from build123d import *

# Parameters (mm, degrees)
PRISM_DEPTH       = 31
CYLINDER030_R     = 2.75
CYLINDER030_DEPTH = 6
CYLINDER029_R     = 5.2188
CYLINDER029_DEPTH = 31
CYLINDER007_R     = 8
CYLINDER007_DEPTH = 1.5
CYLINDER005_R     = 7.5
CYLINDER005_DEPTH = 2
CYLINDER011_R     = 8
CYLINDER011_DEPTH = 1.5
CYLINDER009_R     = 7.5
CYLINDER009_DEPTH = 2
CYLINDER015_R     = 8
CYLINDER015_DEPTH = 1.5
CYLINDER013_R     = 7.5
CYLINDER013_DEPTH = 2
CYLINDER019_R     = 8
CYLINDER019_DEPTH = 1.5
CYLINDER017_R     = 7.5
CYLINDER017_DEPTH = 2
CYLINDER023_R     = 8
CYLINDER023_DEPTH = 1.5
CYLINDER021_R     = 7.5
CYLINDER021_DEPTH = 2
CYLINDER027_R     = 8
CYLINDER027_DEPTH = 1.5
CYLINDER025_R     = 7.5
CYLINDER025_DEPTH = 2
CYLINDER003_R     = 8
CYLINDER003_DEPTH = 1.5
CYLINDER001_R     = 7.5
CYLINDER001_DEPTH = 2
CYLINDER_R        = 9
CYLINDER_DEPTH    = 4


with BuildPart() as prism:
    # prism → prism (new body)
    with BuildSketch(Plane.XY.offset(4)):
        Polygon((5.08068, 0), (2.54034, 4.399998), (-2.54034, 4.399998), (-5.08068, 0), (-2.54034, -4.399998), (2.54034, -4.399998), align=None)
    extrude(amount=PRISM_DEPTH)


with BuildPart() as cylinder030:
    # cylinder030 → cylinder030 (new body)
    with BuildSketch(Plane.XY.offset(-1)):
        Circle(CYLINDER030_R)
    extrude(amount=CYLINDER030_DEPTH)


with BuildPart() as union001:
    # cylinder029 → cylinder029 (new body)
    with BuildSketch(Plane.XY.offset(8)):
        Circle(CYLINDER029_R)
    extrude(amount=CYLINDER029_DEPTH)

    # union001: union prism, cylinder030
    add(prism.part)
    add(cylinder030.part)


with BuildPart() as cylinder006:
    # cylinder006 → cylinder006 (revolve)
    with BuildSketch(Plane(origin=(0, 0, 1.5), x_dir=(1, 0, 0), z_dir=(0, -1, 0))):
        Polygon((0, 0), (7.5, 0), (8, 0.5), (0, 0.5), align=None)
    revolve(axis=Axis((0, 0, 1.5), (0, 0, 1)))


with BuildPart() as cylinder007:
    # cylinder007 → cylinder007 (new body)
    with BuildSketch(Plane.XY.offset(2)):
        Circle(CYLINDER007_R)
    extrude(amount=CYLINDER007_DEPTH)


with BuildPart() as cylinder008:
    # cylinder008 → cylinder008 (revolve)
    with BuildSketch(Plane(origin=(0, 0, 3.5), x_dir=(1, 0, 0), z_dir=(0, -1, 0))):
        Polygon((0, 0), (8, 0), (7.5, 0.5), (0, 0.5), align=None)
    revolve(axis=Axis((0, 0, 3.5), (0, 0, 1)))


with BuildPart() as matrix_union001:
    # cylinder005 → cylinder005 (new body)
    with BuildSketch(Plane.XY):
        Circle(CYLINDER005_R)
    extrude(amount=CYLINDER005_DEPTH)

    # Matrix_Union001: union cylinder006, cylinder007, cylinder008
    add(cylinder006.part)
    add(cylinder007.part)
    add(cylinder008.part)


with BuildPart() as matrix_union001_1:
    # Matrix_Union001 placement: moved
    add(matrix_union001.part.moved(Location((0, 0, 4))))


with BuildPart() as cylinder010:
    # cylinder010 → cylinder010 (revolve)
    with BuildSketch(Plane(origin=(0, 0, 1.5), x_dir=(1, 0, 0), z_dir=(0, -1, 0))):
        Polygon((0, 0), (7.5, 0), (8, 0.5), (0, 0.5), align=None)
    revolve(axis=Axis((0, 0, 1.5), (0, 0, 1)))


with BuildPart() as cylinder011:
    # cylinder011 → cylinder011 (new body)
    with BuildSketch(Plane.XY.offset(2)):
        Circle(CYLINDER011_R)
    extrude(amount=CYLINDER011_DEPTH)


with BuildPart() as cylinder012:
    # cylinder012 → cylinder012 (revolve)
    with BuildSketch(Plane(origin=(0, 0, 3.5), x_dir=(1, 0, 0), z_dir=(0, -1, 0))):
        Polygon((0, 0), (8, 0), (7.5, 0.5), (0, 0.5), align=None)
    revolve(axis=Axis((0, 0, 3.5), (0, 0, 1)))


with BuildPart() as matrix_union002:
    # cylinder009 → cylinder009 (new body)
    with BuildSketch(Plane.XY):
        Circle(CYLINDER009_R)
    extrude(amount=CYLINDER009_DEPTH)

    # Matrix_Union002: union cylinder010, cylinder011, cylinder012
    add(cylinder010.part)
    add(cylinder011.part)
    add(cylinder012.part)


with BuildPart() as matrix_union002_1:
    # Matrix_Union002 placement: moved
    add(matrix_union002.part.moved(Location((0, 0, 8))))


with BuildPart() as cylinder014:
    # cylinder014 → cylinder014 (revolve)
    with BuildSketch(Plane(origin=(0, 0, 1.5), x_dir=(1, 0, 0), z_dir=(0, -1, 0))):
        Polygon((0, 0), (7.5, 0), (8, 0.5), (0, 0.5), align=None)
    revolve(axis=Axis((0, 0, 1.5), (0, 0, 1)))


with BuildPart() as cylinder015:
    # cylinder015 → cylinder015 (new body)
    with BuildSketch(Plane.XY.offset(2)):
        Circle(CYLINDER015_R)
    extrude(amount=CYLINDER015_DEPTH)


with BuildPart() as cylinder016:
    # cylinder016 → cylinder016 (revolve)
    with BuildSketch(Plane(origin=(0, 0, 3.5), x_dir=(1, 0, 0), z_dir=(0, -1, 0))):
        Polygon((0, 0), (8, 0), (7.5, 0.5), (0, 0.5), align=None)
    revolve(axis=Axis((0, 0, 3.5), (0, 0, 1)))


with BuildPart() as matrix_union003:
    # cylinder013 → cylinder013 (new body)
    with BuildSketch(Plane.XY):
        Circle(CYLINDER013_R)
    extrude(amount=CYLINDER013_DEPTH)

    # Matrix_Union003: union cylinder014, cylinder015, cylinder016
    add(cylinder014.part)
    add(cylinder015.part)
    add(cylinder016.part)


with BuildPart() as matrix_union003_1:
    # Matrix_Union003 placement: moved
    add(matrix_union003.part.moved(Location((0, 0, 12))))


with BuildPart() as cylinder018:
    # cylinder018 → cylinder018 (revolve)
    with BuildSketch(Plane(origin=(0, 0, 1.5), x_dir=(1, 0, 0), z_dir=(0, -1, 0))):
        Polygon((0, 0), (7.5, 0), (8, 0.5), (0, 0.5), align=None)
    revolve(axis=Axis((0, 0, 1.5), (0, 0, 1)))


with BuildPart() as cylinder019:
    # cylinder019 → cylinder019 (new body)
    with BuildSketch(Plane.XY.offset(2)):
        Circle(CYLINDER019_R)
    extrude(amount=CYLINDER019_DEPTH)


with BuildPart() as cylinder020:
    # cylinder020 → cylinder020 (revolve)
    with BuildSketch(Plane(origin=(0, 0, 3.5), x_dir=(1, 0, 0), z_dir=(0, -1, 0))):
        Polygon((0, 0), (8, 0), (7.5, 0.5), (0, 0.5), align=None)
    revolve(axis=Axis((0, 0, 3.5), (0, 0, 1)))


with BuildPart() as matrix_union004:
    # cylinder017 → cylinder017 (new body)
    with BuildSketch(Plane.XY):
        Circle(CYLINDER017_R)
    extrude(amount=CYLINDER017_DEPTH)

    # Matrix_Union004: union cylinder018, cylinder019, cylinder020
    add(cylinder018.part)
    add(cylinder019.part)
    add(cylinder020.part)


with BuildPart() as matrix_union004_1:
    # Matrix_Union004 placement: moved
    add(matrix_union004.part.moved(Location((0, 0, 16))))


with BuildPart() as cylinder022:
    # cylinder022 → cylinder022 (revolve)
    with BuildSketch(Plane(origin=(0, 0, 1.5), x_dir=(1, 0, 0), z_dir=(0, -1, 0))):
        Polygon((0, 0), (7.5, 0), (8, 0.5), (0, 0.5), align=None)
    revolve(axis=Axis((0, 0, 1.5), (0, 0, 1)))


with BuildPart() as cylinder023:
    # cylinder023 → cylinder023 (new body)
    with BuildSketch(Plane.XY.offset(2)):
        Circle(CYLINDER023_R)
    extrude(amount=CYLINDER023_DEPTH)


with BuildPart() as cylinder024:
    # cylinder024 → cylinder024 (revolve)
    with BuildSketch(Plane(origin=(0, 0, 3.5), x_dir=(1, 0, 0), z_dir=(0, -1, 0))):
        Polygon((0, 0), (8, 0), (7.5, 0.5), (0, 0.5), align=None)
    revolve(axis=Axis((0, 0, 3.5), (0, 0, 1)))


with BuildPart() as matrix_union005:
    # cylinder021 → cylinder021 (new body)
    with BuildSketch(Plane.XY):
        Circle(CYLINDER021_R)
    extrude(amount=CYLINDER021_DEPTH)

    # Matrix_Union005: union cylinder022, cylinder023, cylinder024
    add(cylinder022.part)
    add(cylinder023.part)
    add(cylinder024.part)


with BuildPart() as matrix_union005_1:
    # Matrix_Union005 placement: moved
    add(matrix_union005.part.moved(Location((0, 0, 20))))


with BuildPart() as cylinder026:
    # cylinder026 → cylinder026 (revolve)
    with BuildSketch(Plane(origin=(0, 0, 1.5), x_dir=(1, 0, 0), z_dir=(0, -1, 0))):
        Polygon((0, 0), (7.5, 0), (8, 0.5), (0, 0.5), align=None)
    revolve(axis=Axis((0, 0, 1.5), (0, 0, 1)))


with BuildPart() as cylinder027:
    # cylinder027 → cylinder027 (new body)
    with BuildSketch(Plane.XY.offset(2)):
        Circle(CYLINDER027_R)
    extrude(amount=CYLINDER027_DEPTH)


with BuildPart() as cylinder028:
    # cylinder028 → cylinder028 (revolve)
    with BuildSketch(Plane(origin=(0, 0, 3.5), x_dir=(1, 0, 0), z_dir=(0, -1, 0))):
        Polygon((0, 0), (8, 0), (7.5, 0.5), (0, 0.5), align=None)
    revolve(axis=Axis((0, 0, 3.5), (0, 0, 1)))


with BuildPart() as matrix_union006:
    # cylinder025 → cylinder025 (new body)
    with BuildSketch(Plane.XY):
        Circle(CYLINDER025_R)
    extrude(amount=CYLINDER025_DEPTH)

    # Matrix_Union006: union cylinder026, cylinder027, cylinder028
    add(cylinder026.part)
    add(cylinder027.part)
    add(cylinder028.part)


with BuildPart() as matrix_union006_1:
    # Matrix_Union006 placement: moved
    add(matrix_union006.part.moved(Location((0, 0, 24))))


with BuildPart() as cylinder002:
    # cylinder002 → cylinder002 (revolve)
    with BuildSketch(Plane(origin=(0, 0, 1.5), x_dir=(1, 0, 0), z_dir=(0, -1, 0))):
        Polygon((0, 0), (7.5, 0), (8, 0.5), (0, 0.5), align=None)
    revolve(axis=Axis((0, 0, 1.5), (0, 0, 1)))


with BuildPart() as cylinder003:
    # cylinder003 → cylinder003 (new body)
    with BuildSketch(Plane.XY.offset(2)):
        Circle(CYLINDER003_R)
    extrude(amount=CYLINDER003_DEPTH)


with BuildPart() as cylinder004:
    # cylinder004 → cylinder004 (revolve)
    with BuildSketch(Plane(origin=(0, 0, 3.5), x_dir=(1, 0, 0), z_dir=(0, -1, 0))):
        Polygon((0, 0), (8, 0), (7.5, 0.5), (0, 0.5), align=None)
    revolve(axis=Axis((0, 0, 3.5), (0, 0, 1)))


with BuildPart() as group003:
    # cylinder001 → cylinder001 (new body)
    with BuildSketch(Plane.XY):
        Circle(CYLINDER001_R)
    extrude(amount=CYLINDER001_DEPTH)

    # Matrix_Union: union cylinder002, cylinder003, cylinder004
    add(cylinder002.part)
    add(cylinder003.part)
    add(cylinder004.part)

    # Group003: union Matrix_Union001, Matrix_Union002, Matrix_Union003, Matrix_Union004, Matrix_Union005, Matrix_Union006
    add(matrix_union001_1.part)
    add(matrix_union002_1.part)
    add(matrix_union003_1.part)
    add(matrix_union004_1.part)
    add(matrix_union005_1.part)
    add(matrix_union006_1.part)


with BuildPart() as group003_1:
    # Group003 placement: moved
    add(group003.part.moved(Location((0, 0, 4))))


with BuildPart() as polebase:
    # cylinder → cylinder (new body)
    with BuildSketch(Plane.XY):
        Circle(CYLINDER_R)
    extrude(amount=CYLINDER_DEPTH)

    # union: union Group003
    add(group003_1.part)

    # difference: cut union001
    add(union001.part, mode=Mode.SUBTRACT)


solid = polebase.part
Check sheet for the modelled part. Datum: model origin and axes. Units: mm. A direction names the side the tool comes from. Round coordinates to 2 decimals unless told otherwise and drop trailing zeros. Loops run counter-clockwise (first coordinate to the right, second up) from the corner with the lowest first, then second, coordinate; pieces in that order, holes last.
1. Gauge pin test, flat ends, axial feed: pin 1 Ø5 at (y, z) = (-6.5, 26.5) entering from -X; pin 2 Ø5.5 at (x, y) = (-1.5, -2.5) entering from +Z; pin 3 Ø10 at (y, z) = (2.5, 28) entering from -X; pin 4 Ø5 at (x, z) = (5.5, 12.5) entering from -Y. Record the tip position at first contact, or that the pin passes through.
2. Set-up check for faces 4 (the cylindrical face through (-7.493, 0.33, 20.74)), 5 (the cylindrical face through (4.978, 1.568, 19.832)), 6 (the flat face through (2, 5, 32)): record each of +Z, -Z, +X, -X, +Y, -Y from which the full face is reachable in a straight line by a thin tool's end or side.
3. Scan lines: probe 1 along Y at (x, z) = (0, 14.25); probe 2 along Z at (x, y) = (-6, 6); probe 3 along Y at (x, z) = (3.25, 15). Record each from-to range of solid material in increasing order.
4. Sectioned sample at B-B on z = 28.5. Record the boundary of the cut face in (x, y).
5. Sectioned sample at A-A on z = 4.5. Record the boundary of the cut face in (x, y), and give its area (3 significant figures).
6. Mould release check, pull along Z, two halves, no side actions. Record for faces 1 (the flat face through (0, -5, 8)), 2 (the cylindrical face through (-1.73, -7.81, 10.74)), 3 (the cylindrical face through (-7.493, 0.33, 8.74)): released by +Z, released by -Z, zero draft, split by the parting line, or undercut.
Recorded:
1. pin 1: stops at x = -6.93
1. pin 2: stops at z = 32
1. pin 3: stops at x = -8
1. pin 4: stops at y = -7.33
2. face 4: none
2. face 5: +Z
2. face 6: +Z, +X, -X, +Y, -Y
3. probe 1: y = -8 to -5.22, 5.22 to 8
3. probe 2: z = 0 to 4
3. probe 3: y = -7.31 to -4.08, 4.08 to 7.31
4. outline: circle Ø15 at (0, 0); hole circle Ø10.44 at (0, 0)
5. outline: circle Ø15 at (0, 0); hole (-5.08, 0) - (-2.54, -4.4) - (2.54, -4.4) - (5.08, 0) - (2.54, 4.4) - (-2.54, 4.4) - close
5. area: 110 mm2
6. face 1: released by +Z
6. face 2: zero draft
6. face 3: undercut
